from build123d import *

# Parameters (mm, degrees)
F0_W     = 100
F0_H     = 50
F1_DEPTH = 40
F2_T     = -2.5
F4_DEPTH = 50


with BuildPart() as f1:
    # F0 (on Top) → F1 (new body)
    with BuildSketch(Plane.XY):
        Rectangle(F0_W, F0_H)
    extrude(amount=-F1_DEPTH)

    # F2
    f2_openings = [f1.faces().sort_by_distance(p)[0] for p in [
        (0, 0, 0),
    ]]
    offset(amount=F2_T, openings=f2_openings)

    # F3 (on Right) → F4 (join, symmetric)
    with BuildSketch(Plane.YZ):
        with BuildLine():
            Line((-25, 0), (25, 0))
            ThreePointArc((25, 0), (0, 25), (-25, 0))
        make_face()
    extrude(amount=F4_DEPTH, both=True)


solid = f1.part
The model under review builds one solid part; all positions refer to its coordinate system, in mm. A direction names the side the tool comes from. Round coordinates to 2 decimals unless told otherwise and drop trailing zeros. Write each loop counter-clockwise with the first axis right and the second up, starting at its lowest first coordinate (ties: lowest second). Pieces come first, ordered by that corner, then holes. Notation, with made-up numbers: (59, 82.5) - (116, 82.5) arc R24 ccw to (116, 101.5) - close; hole circle Ø8 at (29, 57). An arc over 180 degrees is marked (long way). One line per item, written item: value. Start each with the question number.
1. The part is to be moulded in two halves that separate along X. For faces 3 (the face through (-47.5, 0, -18)), 4 (the face through (0.7, 0.55, 24.994)), 5 (the face through (50, 0, -7)), say which applies: released by +X, released by -X, zero draft, split by the parting line, or undercut.
2. Clearance check with flat-ended pins moving along their axes: P1, Ø12, axis at x = -24.5, y = 16, coming from the +Z side; P2, Ø2, axis at x = -21, z = 2, coming from the +Y side; P3, Ø2, axis at x = 2.5, z = 18, coming from the +Y side. State where each tip first meets the part, or that it passes through.
3. To check wall thickness, follow L1, parallel to Y at x = 44, z = -3.5; L2, parallel to X at y = -8.5, z = -34; L3, parallel to Z at x = 3, y = -20. State the ranges of each line that lie inside material, in increasing order. Write a range as from..to.
4. Machinability: for faces 1 (the face through (-50, 0, -7)), 2 (the face through (-1, 0, -37.5)), which of the approach directions +Z, -Z, +X, -X, +Y, -Y give a long, thin tool a straight path to every point of the face, cutting with its end or side? Answer none if there is none.
5. Consider section A-A on z = -13. Write out the cut boundary in (x, y).
6. Consider section B-B on y = -15. Write out the cut boundary in (x, z).
7. Consider section D-D on z = 6.5. Write out the cut boundary in (x, y), and give its area (3 significant figures).
8. Consider section C-C on z = 17. Write out the cut boundary in (x, y), and give its area (3 significant figures).
Checks:
1. face 3: undercut
1. face 4: zero draft
1. face 5: released by +X
2. P1: stops at z = 22.91
2. P2: stops at y = 24.98
2. P3: stops at y = 18.33
3. L1: y = -25..-22.5, 22.5..25
3. L2: x = -50..-47.5, 47.5..50
3. L3: z = -40..-37.5, 0..15
4. face 1: +Z, -Z, -X, +Y, -Y
4. face 2: none
5. outline: (-50, -25) - (50, -25) - (50, 25) - (-50, 25) - close; hole (-47.5, -22.5) - (47.5, -22.5) - (47.5, 22.5) - (-47.5, 22.5) - close
6. outline: (-50, -40) - (50, -40) - (50, 20) - (-50, 20) - close; hole (-47.5, -37.5) - (47.5, -37.5) - (47.5, 0) - (-47.5, 0) - close
7. outline: (-50, -24.14) - (50, -24.14) - (50, 24.14) - (-50, 24.14) - close
7. area: 4,830 mm^2
8. outline: (-50, -18.33) - (50, -18.33) - (50, 18.33) - (-50, 18.33) - close
8. area: 3,670 mm^2
